The listing builds one solid part. Answer for the finished solid, in the listing's coordinates (mm). Coordinates: 2 decimals unless noted, no trailing zeros. Order: outer loops, then holes, each group sorted by start corner. A loop starts at its lowest first (then second) coordinate and runs counter-clockwise, first axis right, second up. Notation, with made-up numbers: (79.25, -4.75) -> (110.25, -4.75) arc R15 cw to (110.25, -0.75) -> close; hole circle Ø4 at (48, 38). An arc over 180 degrees is marked (long way). One line per question, with ' | ' between items.
from build123d import *

# Parameters (mm, degrees)
BOSS_EXTRUDE1_DEPTH = 2
SKETCH2_R           = 2
BOSS_EXTRUDE2_DEPTH = 2


with BuildPart() as part:
    # Sketch1 → Boss-Extrude1 (new body)
    with BuildSketch(Plane(origin=(0, 0, 0), x_dir=(1, 0, 0), z_dir=(0, 1, 0))):
        with BuildLine():
            Line((-10, 17.75), (19, 17.75))
            Line((19, 17.75), (19, -17.75))
            Line((19, -17.75), (-10, -17.75))
            ThreePointArc((-10, -17.75), (-16.363961031, -15.113961031), (-19, -8.75))
            Line((-19, -8.75), (-19, 8.75))
            ThreePointArc((-19, 8.75), (-16.363961031, 15.113961031), (-10, 17.75))
        make_face()
    extrude(amount=BOSS_EXTRUDE1_DEPTH)

    # Sketch2 → Boss-Extrude2 (add)
    with BuildSketch(Plane(origin=(0, 0, -17.75), x_dir=(-1, 0, 0), z_dir=(0, 0, -1))):
        with BuildLine():
            Line((-10.5, 0), (-13.689709334, -2.577891806))
            ThreePointArc((-13.689709334, -2.577891806), (-14.346103242, -8.765714286), (-8.158280763, -9.422108194))
            Line((-8.158280763, -9.422108194), (3.5, 0))
            Line((3.5, 0), (-10.5, 0))
        make_face()
        with Locations((-10.923995048, -6)):
            Circle(SKETCH2_R, mode=Mode.SUBTRACT)
    extrude(amount=-BOSS_EXTRUDE2_DEPTH)


solid = part.part
Item 1: Section D-D, the plane z = -8 is taken. Give the vertices of the cut face in (x, y), plus the area to 3 significant figures.
Computed values:
outline: (-19, 0) -> (19, 0) -> (19, 2) -> (-19, 2) -> close | area: 76.0 mm^2
Item 2: Section A-A, the plane y = -5 is taken. Give the vertices of the cut face in (x, z).
Computed values:
outline: (2.69, -17.75) -> (9.19, -17.75) -> (9.19, -15.75) -> (2.69, -15.75) -> close; (12.66, -17.75) -> (15.21, -17.75) -> (15.21, -15.75) -> (12.66, -15.75) -> close
Item 3: Determine the mould class of faces 1 (the face through (12.07, -1.27, -16.76)), 2 (the face through (0, 2, 0)), 3 (the face through (8, -4, -15.75)) for opening direction Y: pulls with the +Y half, pulls with the -Y half, needs draft (parallel to the pull), parting line crosses it, or undercut.
Computed values:
face 1: undercut | face 2: pulls with the +Y half | face 3: needs draft
Item 4: Find the intervals of material crossed by L1, parallel to Y at x = 14.5, z = 8.5; L2, parallel to Z at x = 9.5, y = -9.5; L3, parallel to X at y = -6.25, z = -16, in increasing order.
Computed values:
L1: y = 0 to 2 | L2: z = -17.75 to -15.75 | L3: x = 4.23 to 8.94, 12.91 to 15.32
Item 5: Section B-B, the plane y = 0.5 is taken. Give the vertices of the cut face in (x, z), plus the area to 3 significant figures.
Computed values:
outline: (-19, -8.75) arc R9 ccw to (-10, -17.75) -> (19, -17.75) -> (19, 17.75) -> (-10, 17.75) arc R9 ccw to (-19, 8.75) -> close | area: 1,310 mm^2
Item 6: Section C-C, the plane x = 3 is taken. Give the vertices of the cut face in (y, z).
Computed values:
outline: (-5.25, -17.75) -> (2, -17.75) -> (2, 17.75) -> (0, 17.75) -> (0, -15.75) -> (-5.25, -15.75) -> close
Item 7: Each of these flat-tipped pins is pushed along its axis until it touches: pin 1 Ø4.5 at (x, y) = (10.92, -6) entering from +Z; pin 2 Ø8 at (x, z) = (-6, 8.5) entering from -Y; pin 3 Ø6 at (x, y) = (12.5, -5) entering from -Z. Where does it stop, or does it pass through?
Computed values:
pin 1: stops at z = -15.75 | pin 2: stops at y = 0 | pin 3: stops at z = -17.75
